Read the model definition and answer for the solid it produces. Units are mm, in the model's axes. A direction names the side the tool comes from. Give positions to 0.01 mm unless a question says otherwise; leave off trailing zeros. Order: outer loops, then holes, each group sorted by start corner. A loop starts at its lowest first (then second) coordinate and runs counter-clockwise, first axis right, second up. Notation, with made-up numbers: (-7, -31.5) - (26, -31.5) arc R16 ccw to (26, -22.5) - close; hole circle Ø1 at (20, -34.5). An arc over 180 degrees is marked (long way). Use a Markdown table: item, result. Add a question column.
1. A cutting plane is placed at A-A on y = 44.5. Determine the outline of the cut face in (x, z).
2. For a pull along X with two mould halves and no side action, classify faces 4 (the flat face through (0.1, 98.5, 4.3)), 5 (the cylindrical face through (2.285, 18.127, -3.584)), 6 (the conical face through (0.16, 37.11, 0.72)), 7 (the cylindrical face through (5, 109, 0)) as released by +X, released by -X, zero draft, split by the parting line, or undercut.
3. Flat-ended cylindrical pins translate along their axes: P1, Ø10, axis at x = 7.5, y = 100, coming from the -Z side; P2, Ø1.5, axis at y = 58.5, z = -4.5, coming from the +X side; P3, Ø3, axis at x = 4.5, y = 63, coming from the +Z side. Find the tip coordinate at first contact, or state that the pin passes through.
4. Consider L1, parallel to Z at x = 0, y = 10.5; L2, parallel to Y at x = -6, z = 6.25; L3, parallel to Y at x = 0.5, z = -9. Determine where each line is inside the solid, lowest interval first.
5. Which of the six approach directions +Z, -Z, +X, -X, +Y, -Y give full straight-line access (tool end or side, diameter ignored) to faces 1 (the flat face through (0, 10, 8.5)), 2 (the flat face through (0, 10, -8.5)), 3 (the flat face through (0, 109, 4))?
```python
from build123d import *

# Parameters (mm, degrees)
ESQUISSE1_R                  = 10
BOSS_EXTRU_1_DEPTH           = 120
ESQUISSE2_R                  = 10
ESQUISSE2_R_2                = 5
ENL_V_MAT_EXTRU_1_DEPTH      = 21.5
TROU_TARAUD_M101_D           = 8.5
TROU_TARAUD_M101_DEPTH       = 35
TROU_TARAUD_M101_CSINK_D     = 10.05
TROU_TARAUD_M101_CSINK_ANGLE = 90
TROU_TARAUD_M101_TIP         = 2.553657631
ESQUISSE14_W                 = 20
ESQUISSE14_H                 = 1.5
ENL_V_MAT_EXTRU_2_DEPTH      = 20
ESQUISSE15_W                 = 20
ESQUISSE15_H                 = 1
ENL_V_MAT_EXTRU_5_DEPTH      = 21.5


with BuildPart() as part:
    # Esquisse1 → Boss.-Extru.1 (new body)
    with BuildSketch(Plane(origin=(0, 0, 0), x_dir=(1, 0, 0), z_dir=(0, 1, 0))):
        with Locations(Location((0, 0, 0), (0, 0, 270))):  # turned: the seam where the file's is
            Circle(ESQUISSE1_R)
    extrude(amount=BOSS_EXTRU_1_DEPTH)

    # Esquisse2 → Enlèv. mat.-Extru.1 (cut)
    with BuildSketch(Plane(origin=(0, 120, 0), x_dir=(1, 0, 0), z_dir=(0, 1, 0))):
        with Locations(Location((0, 0, 0), (0, 0, 270))):  # turned: the seam where the file's is
            Circle(ESQUISSE2_R)
        with Locations(Location((0, 0, 0), (0, 0, 270))):  # turned: the seam where the file's is
            Circle(ESQUISSE2_R_2, mode=Mode.SUBTRACT)
    extrude(amount=-ENL_V_MAT_EXTRU_1_DEPTH, mode=Mode.SUBTRACT)

    # Trou taraudé M101
    with Locations(Plane(origin=(0, 0, 0), x_dir=(-1, 0, 0), z_dir=(0, -1, 0))):
        with Locations((0, 0)):
            CounterSinkHole(TROU_TARAUD_M101_D / 2, TROU_TARAUD_M101_CSINK_D / 2, depth=TROU_TARAUD_M101_DEPTH, counter_sink_angle=TROU_TARAUD_M101_CSINK_ANGLE)
            with Locations((0, 0, -(TROU_TARAUD_M101_DEPTH + TROU_TARAUD_M101_TIP / 2))):  # 118° drill point
                Cone(0, TROU_TARAUD_M101_D / 2, TROU_TARAUD_M101_TIP, mode=Mode.SUBTRACT)

    # Esquisse14 → Enlèv. mat.-Extru.2 (cut)
    with BuildSketch(Plane.XZ):
        with Locations((0, 9.25)):
            Rectangle(ESQUISSE14_W, ESQUISSE14_H)
        with Locations((0, -9.25)):
            Rectangle(ESQUISSE14_W, ESQUISSE14_H)
    extrude(amount=-ENL_V_MAT_EXTRU_2_DEPTH, mode=Mode.SUBTRACT)

    # Esquisse15 → Enlèv. mat.-Extru.5 (cut)
    with BuildSketch(Plane(origin=(0, 120, 0), x_dir=(1, 0, 0), z_dir=(0, 1, 0))):
        with Locations((0, 4.5)):
            Rectangle(ESQUISSE15_W, ESQUISSE15_H)
        with Locations((0, -4.5)):
            Rectangle(ESQUISSE15_W, ESQUISSE15_H)
    extrude(amount=-ENL_V_MAT_EXTRU_5_DEPTH, mode=Mode.SUBTRACT)


solid = part.part
```
Output values:
| question | item | result |
|---|---|---|
| 1 | outline | circle Ø20 at (0, 0) |
| 2 | face 4 | zero draft |
| 2 | face 5 | undercut |
| 2 | face 6 | undercut |
| 2 | face 7 | released by +X |
| 3 | P1 | z = -9.62 |
| 3 | P2 | x = 9.27 |
| 3 | P3 | z = 9.54 |
| 4 | L1 | -8.5 to -4.25, 4.25 to 8.5 |
| 4 | L2 | 0 to 98.5 |
| 4 | L3 | 20 to 98.5 |
| 5 | face 1 | +Z, +X, -X, -Y |
| 5 | face 2 | -Z, +X, -X, -Y |
| 5 | face 3 | +Z, +X, -X, +Y |
